Check sheet for the modelled part. Datum: model origin and axes. Units: mm. A direction names the side the tool comes from. Coordinates: 2 decimals unless noted, no trailing zeros. Write each loop counter-clockwise with the first axis right and the second up, starting at its lowest first coordinate (ties: lowest second). Pieces come first, ordered by that corner, then holes. Notation, with made-up numbers: (-13, 69.5) -> (39, 69.5) arc R23 cw to (39, 79.5) -> close; hole circle Ø4 at (-21, -40). An arc over 180 degrees is marked (long way). Put each result on its own line as item: value.
```python
from build123d import *
from OCP.BRepFilletAPI import BRepFilletAPI_MakeChamfer

# Parameters (mm, degrees)
BOSS_EXTRUDE1_DEPTH = 2
BOSS_EXTRUDE2_DEPTH = 25
BOSS_EXTRUDE3_DEPTH = 10
CUT_EXTRUDE4_DEPTH  = 2
CUT_EXTRUDE5_DEPTH  = 2
CUT_EXTRUDE6_DEPTH  = 2
CUT_EXTRUDE7_DEPTH  = 2
CHAMFER1_SIZE       = 0.727940469
CHAMFER1_SIZE_2     = 2
CHAMFER2_SIZE       = 2
CHAMFER2_SIZE2      = 1.72643598


with BuildPart() as part:
    # Sketch12 → Boss-Extrude1 (new body)
    with BuildSketch(Plane(origin=(0, 0, 0), x_dir=(1, 0, 0), z_dir=(0, 1, 0))):
        Polygon((-27, -6.414360409), (-27, -2.352653961), (-25, -2), (25, -2), (27, -2.352653961), (27, -6.414360409), (35.023054857, -7.829041448), (35.023054857, -1.736481777), (25.174977327, 0), (-25.174977327, 0), (-35.023054857, -1.736481777), (-35.023054857, -7.829041448), align=None)
    extrude(amount=BOSS_EXTRUDE1_DEPTH)

    # Sketch13 → Boss-Extrude2 (add)
    with BuildSketch(Plane.XZ):
        Polygon((25.174977327, 0), (35.023054857, 1.736481777), (35.023054857, 3.767335), (27, 2.352653961), (25, 2), (-25, 2), (-27, 2.352653961), (-35.023054857, 3.767335), (-35.023054857, 1.736481777), (-25.174977327, 0), align=None)
    extrude(amount=BOSS_EXTRUDE2_DEPTH)

    # Sketch14 → Boss-Extrude3 (add)
    with BuildSketch(Plane.XZ):
        Polygon((-35.023054857, 7.829041448), (-27, 6.414360409), (-27, 4.383507185), (-35.023054857, 5.798188224), align=None)
        Polygon((27, 6.414360409), (35.023054857, 7.829041448), (35.023054857, 5.798188224), (27, 4.383507185), align=None)
    extrude(amount=BOSS_EXTRUDE3_DEPTH)

    # Sketch15 → Cut-Extrude4 (cut)
    with BuildSketch(Plane(origin=(0.759118452, 0, -4.305174677), x_dir=(-0.9848077530121055, 0, -0.1736481776675121), z_dir=(0.1736481776675121, 0, -0.9848077530121055))):
        Polygon((-24.792512854, -25), (-35.145166815, -14.647346039), (-35.145166815, -25), align=None)
    extrude(amount=-CUT_EXTRUDE4_DEPTH, mode=Mode.SUBTRACT)

    # Sketch16 → Cut-Extrude5 (cut)
    with BuildSketch(Plane(origin=(-0.759118452, 0, -4.305174677), x_dir=(-0.9848077530121054, 0, 0.17364817766751298), z_dir=(-0.17364817766751298, 0, -0.9848077530121054))):
        Polygon((24.792512854, -25), (35.145166815, -14.647346039), (35.145166815, -25), align=None)
    extrude(amount=-CUT_EXTRUDE5_DEPTH, mode=Mode.SUBTRACT)

    # Sketch18 → Cut-Extrude6 (cut)
    with BuildSketch(Plane(origin=(0.282770614, 0, 1.603671841), x_dir=(0.9848077530121053, 0, -0.17364817766751298), z_dir=(0.173648177667513, 0, 0.9848077530121054))):
        Polygon((-31.777063033, -10), (-35.850474738, -4), (-35.850474738, -10), align=None)
    extrude(amount=-CUT_EXTRUDE6_DEPTH, mode=Mode.SUBTRACT)

    # Sketch19 → Cut-Extrude7 (cut)
    with BuildSketch(Plane(origin=(-0.282770614, 0, 1.603671841), x_dir=(0.9848077530121055, 0, 0.17364817766751214), z_dir=(-0.17364817766751214, 0, 0.9848077530121055))):
        Polygon((31.777063033, -10), (35.850474738, -4), (35.850474738, -10), align=None)
    extrude(amount=-CUT_EXTRUDE7_DEPTH, mode=Mode.SUBTRACT)

    # Chamfer1
    chamfer1_edges_1 = [part.edges().sort_by_distance(p)[0] for p in [
        (-35.023054857, 2, 4.782761612),
    ]]
    chamfer1_side_1 = [part.faces().sort_by_distance(p)[0] for p in [
        (-35.008496048, 2, 4.782761612),
    ]]
    chamfer1_edges_2 = [part.edges().sort_by_distance(p)[0] for p in [
        (35.023054857, 2, 4.782761612),
    ]]
    chamfer1_side_2 = [part.faces().sort_by_distance(p)[0] for p in [
        (35.008496048, 2, 4.782761612),
    ]]
    chamfer1 = BRepFilletAPI_MakeChamfer(part.part.solid().wrapped)
    for e in chamfer1_edges_1:
        chamfer1.Add(CHAMFER1_SIZE - 0.0001, CHAMFER1_SIZE_2 - 0.0001, e.wrapped, chamfer1_side_1[0].wrapped)
    for e in chamfer1_edges_2:
        chamfer1.Add(CHAMFER1_SIZE - 0.0001, CHAMFER1_SIZE_2 - 0.0001, e.wrapped, chamfer1_side_2[0].wrapped)
    add(Compound.cast(chamfer1.Shape()), mode=Mode.REPLACE)  # a hair under: the kernel refuses the full size

    # Chamfer2: one chamfer whose edges measure the first distance from different faces: ONE call of the kernel's chamfer builder (chamfer() names one face for all edges)
    chamfer2_edges_1 = [part.edges().sort_by_distance(p)[0] for p in [
        (-35.023054857, -1.99995, 7.829041448),
    ]]
    chamfer2_side_1 = [part.faces().sort_by_distance(p)[0] for p in [
        (-35.023054857, -6.233576758, 3.65083088),
    ]]
    chamfer2_edges_2 = [part.edges().sort_by_distance(p)[0] for p in [
        (35.023054857, -1.99995, 7.829041448),
    ]]
    chamfer2_side_2 = [part.faces().sort_by_distance(p)[0] for p in [
        (30.593302678, -3.470070419, 7.047956621),
    ]]
    chamfer2 = BRepFilletAPI_MakeChamfer(part.part.solid().wrapped)
    for e in chamfer2_edges_1:
        chamfer2.Add(CHAMFER2_SIZE, CHAMFER2_SIZE2, e.wrapped, chamfer2_side_1[0].wrapped)  # the first distance lies on this face
    for e in chamfer2_edges_2:
        chamfer2.Add(CHAMFER2_SIZE, CHAMFER2_SIZE2, e.wrapped, chamfer2_side_2[0].wrapped)  # the first distance lies on this face
    add(Compound.cast(chamfer2.Shape()), mode=Mode.REPLACE)


solid = part.part
```
Q1. Cross-section at A-A (y = -1.5). State how many separate pieces and enclosed holes the cut face has, plus the area to 3 significant figures.
Recorded:
separate pieces: 3
enclosed holes: 0
area: 170 mm2
Q2. Material ranges on line 1 along Z through (x, y) = (14, -20.25); line 2 along X through (y, z) = (-8, 6); line 3 along Y through (x, z) = (28, 6.5), recorded low to high.
Recorded:
line 1: z = 0 to 2
line 2: x = -32.59 to -27, 27 to 32.59
line 3: y = -10 to 2
Q3. Mould release check, pull along X, two halves, no side actions. Record for faces 4 (the flat face through (29, -10, 6)), 5 (the flat face through (-31, 0, 4)), 6 (the flat face through (31.07, -4.93, 5.1)): released by +X, released by -X, zero draft, split by the parting line, or undercut.
Recorded:
face 4: zero draft
face 5: undercut
face 6: released by +X
Q4. Depth check by flat-ended pin: P1, Ø0.8, axis at x = -29, z = 6, coming from the -Y side; P2, Ø13.5, axis at x = 2, y = -5, coming from the +Z side; P3, Ø4, axis at x = -29.5, z = 4.5, coming from the -Y side. Enter the tip coordinate at first touch or a pass-through.
Recorded:
P1: stops at y = -10
P2: stops at z = 2
P3: stops at y = -21.04
Q5. Tool access check on faces 1 (the flat face through (29.98, -4.08, 6.94)), 2 (the flat face through (-30.96, -4.93, 5.08)), 3 (the flat face through (-30.17, -8.31, 0.88)). Record the directions out of +Z, -Z, +X, -X, +Y, -Y that give a thin tool (end or side, any length) a straight path to the whole face; none if there is none.
Recorded:
face 1: +Z, +Y, -Y
face 2: -X, -Y
face 3: -Z, -X, +Y, -Y
Q6. Cross-section at D-D (x = 4.5). Record the cut outline in (y, z), plus the area to 3 significant figures.
Recorded:
outline: (-25, 0) -> (2, 0) -> (2, 2) -> (-25, 2) -> close
area: 54.0 mm2
Q7. Cross-section at B-B (z = 3). Record the cut outline in (x, y).
Recorded:
outline: (-35.02, -14.78) -> (-30.67, -19.07) -> (-30.67, 0) -> (-27, 0) -> (-27, 2) -> (-34.3, 2) -> (-35.02, 0) -> close; (27, 0) -> (30.67, 0) -> (30.67, -19.07) -> (35.02, -14.78) -> (35.02, 0) -> (34.3, 2) -> (27, 2) -> close
Q8. Cross-section at C-C (y = -12). Record the cut outline in (x, z).
Recorded:
outline: (-35.02, 1.74) -> (-25.17, 0) -> (25.17, 0) -> (35.02, 1.74) -> (35.02, 3.77) -> (25, 2) -> (-25, 2) -> (-35.02, 3.77) -> close
